Check sheet for the modelled part. Datum: model origin and axes. Units: mm. Face numbers are marked on the shaded views. Round coordinates to 2 decimals unless told otherwise and drop trailing zeros. Loops run counter-clockwise (first coordinate to the right, second up) from the corner with the lowest first, then second, coordinate; pieces in that order, holes last. Notation, with made-up numbers: (-26, 13.5) -> (-6, 13.5) arc R19 ccw to (-6, 37.5) -> close; hole circle Ø6 at (-23.5, 73). An arc over 180 degrees is marked (long way). Use one line per item in the form item = value. Start each with the question number.
(1) Sectioned sample at C-C (z = 4.25). Record the cut outline in (x, y), and give its area (3 significant figures).
(2) Draft check along Y on the marked faces 1 and 2. Enter one of: released by +Y, released by -Y, zero draft, split by the parting line, or undercut.
(3) Material ranges on probe 1 along Y at (x, z) = (0, 4.5); probe 2 along X at (y, z) = (1.5, 0.5); probe 3 along X at (y, z) = (5, 1.5), recorded low to high. Write a range as [from, to].
(4) Go/stop test with flat-tipped pins: pin 1 (5 mm diameter, centred on y = 3, z = 2, fed in from +X); pin 2 (1 mm diameter, centred on x = -9.5, z = 5, fed in from +Y); pin 3 (4 mm diameter, centred on y = 6, z = 1, fed in from -X). Record where each tip stops, or that it passes through.
(5) Sectioned sample at A-A (x = 0). Record the cut outline in (y, z), and give its area (3 significant figures).
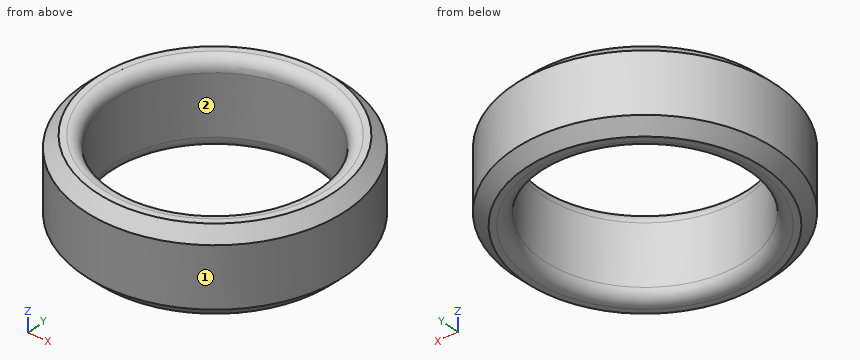
from build123d import *

# Parameters (mm, degrees)
F0_R     = 13.97
F0_R_2   = 10.7696
F1_DEPTH = 8.89
F2_R     = 1.27
F3_SIZE  = 1.27


with BuildPart() as f1:
    # F0 (on Top) → F1 (new body)
    with BuildSketch(Plane.XY):
        Circle(F0_R)
        Circle(F0_R_2, mode=Mode.SUBTRACT)
    extrude(amount=F1_DEPTH)

    # F2
    f2_edges = [f1.edges().sort_by_distance(p)[0] for p in [
        (-10.7696, 0, 8.89),
        (-10.7696, 0, 0),
    ]]
    fillet(f2_edges, radius=F2_R)

    # F3
    f3_edges = [f1.edges().sort_by_distance(p)[0] for p in [
        (13.97, 0, 4.445),
        (-13.97, 0, 0),
        (-13.97, 0, 8.89),
    ]]
    chamfer(f3_edges, length=F3_SIZE)


solid = f1.part
Checks:
q1.outline = circle Ø27.94 at (0, 0); hole circle Ø21.54 at (0, 0)
q1.area = 249 mm2
q2.face_1 = split by the parting line
q2.face_2 = undercut
q3.probe_1 = [-13.97, -10.77], [10.77, 13.97]
q3.probe_2 = [-13.11, -10.93], [10.93, 13.11]
q3.probe_3 = [-13.04, -9.54], [9.54, 13.04]
q4.pin_1 = 13.96
q4.pin_2 = 10.68
q4.pin_3 = -13.38
q5.outline = (-13.97, 1.27) -> (-12.7, 0) -> (-12.04, 0) arc R1.27 ccw to (-10.77, 1.27) -> (-10.77, 7.62) arc R1.27 ccw to (-12.04, 8.89) -> (-12.7, 8.89) -> (-13.97, 7.62) -> close; (10.77, 1.27) arc R1.27 ccw to (12.04, 0) -> (12.7, 0) -> (13.97, 1.27) -> (13.97, 7.62) -> (12.7, 8.89) -> (12.04, 8.89) arc R1.27 ccw to (10.77, 7.62) -> close
q5.area = 52.3 mm2
